from build123d import *

# Parameters (mm, degrees)
SKETCH_1_W          = 15.2
SKETCH_1_H          = 25
EXTRUDE_1_DEPTH     = 3
EXTRUDE_3_DEPTH     = 10
EXTRUDE_4_DEPTH     = 25
CUT_EXTRUDE_1_DEPTH = 18
FILLET_2_R          = 2
CHAMFER_1_SIZE      = 1
CHAMFER_2_SIZE      = 0.4


with BuildPart() as part:
    # 草图1 → 凸台-拉伸1 (new body)
    with BuildSketch(Plane(origin=(0, 0, 0), x_dir=(1, 0, 0), z_dir=(0, 1, 0))):
        Rectangle(SKETCH_1_W, SKETCH_1_H)
    extrude(amount=EXTRUDE_1_DEPTH)

    # 草图4 → 凸台-拉伸3 (add)
    with BuildSketch(Plane.ZY.offset(7.6)):
        Polygon((-12.5, -15), (-12.5, 3), (12.5, 3), (12.5, 0), align=None)
    extrude_3 = extrude(amount=EXTRUDE_3_DEPTH)

    # 镜向4: 凸台-拉伸3 across plane
    add(extrude_3.mirror(Plane(origin=(0, 0, 0), x_dir=(0, 0, 1), z_dir=(1, 0, 0))))

    # 草图5 → 凸台-拉伸4 (add)
    with BuildSketch(Plane(origin=(0, 0, -12.5), x_dir=(-1, 0, 0), z_dir=(0, 0, -1))):
        Polygon((7.6, 0), (7.6, -15), (17.6, -15), (17.6, 3), (-17.6, 3), (-17.6, -15), (-7.6, -15), (-7.6, 0), align=None)
    extrude(amount=EXTRUDE_4_DEPTH)

    # 草图6 → 切除-拉伸1 (cut)
    with BuildSketch(Plane(origin=(0, 3, 0), x_dir=(1, 0, 0), z_dir=(0, 1, 0))):
        Polygon((14.072075922, 37.6), (10.927924078, 37.6), (9.861257411, 34.4), (15.138742589, 34.4), align=None)
        Polygon((-14.072075922, 37.6), (-15.138742589, 34.4), (-9.861257411, 34.4), (-10.927924078, 37.6), align=None)
    extrude(amount=-CUT_EXTRUDE_1_DEPTH, mode=Mode.SUBTRACT)

    # 圆角2
    fillet_2_edges = [part.edges().sort_by_distance(p)[0] for p in [
        (-12.6, -15, -12.5),
        (12.6, -15, -12.5),
    ]]
    fillet(fillet_2_edges, radius=FILLET_2_R)

    # 倒角1
    chamfer_1_edges = [part.edges().sort_by_distance(p)[0] for p in [
        (-7.6, -7.357492926, 0.23751179),
        (-17.6, -7.357492926, 0.23751179),
        (-7.6, -14.927429856, -12.520100766),
        (-17.6, -14.927429856, -12.520100766),
        (7.6, -7.357492926, 0.23751179),
        (7.6, -14.927429856, -12.520100766),
        (17.6, -7.357492926, 0.23751179),
        (17.6, -14.927429856, -12.520100766),
        (-17.6, 1.5, 12.5),
        (-17.6, 3, -12.5),
        (17.6, 3, -12.5),
        (17.6, 1.5, 12.5),
        (7.6, -15, -25.276983965),
        (-7.6, -15, -25.276983965),
        (-17.6, -15, -25.276983965),
        (17.6, -15, -25.276983965),
        (7.6, -7.5, -37.5),
        (-7.6, -7.5, -37.5),
        (-17.6, -6, -37.5),
        (17.6, -6, -37.5),
    ]]
    chamfer(chamfer_1_edges, length=CHAMFER_1_SIZE)

    # 倒角2
    chamfer_2_edges = [part.edges().sort_by_distance(p)[0] for p in [
        (10.377924078, 3, -35.95),
        (12.5, 3, -34.4),
        (14.622075922, 3, -35.95),
        (14.622075922, -15, -35.95),
        (12.5, -15, -34.4),
        (10.377924078, -15, -35.95),
        (-14.622075922, 3, -35.95),
        (-12.5, 3, -34.4),
        (-10.377924078, 3, -35.95),
        (-10.377924078, -15, -35.95),
        (-12.5, -15, -34.4),
        (-14.622075922, -15, -35.95),
    ]]
    chamfer(chamfer_2_edges, length=CHAMFER_2_SIZE)


solid = part.part
Design review of the part built by this model. Coordinates are the model's own, in mm. A direction names the side the tool comes from. Give positions to 0.01 mm unless a question says otherwise; leave off trailing zeros. Write each loop counter-clockwise with the first axis right and the second up, starting at its lowest first coordinate (ties: lowest second). Pieces come first, ordered by that corner, then holes. Notation, with made-up numbers: M 80,59 L 103,59 A16 cw 103,80 Z; hole C 21,-7.5 d3. An arc over 180 degrees is marked long. Answer as a JSON object with one key per item and string values. Group by question number.
1) Mouldability with a two-part tool opening along X and no side actions: class faces 1 (the face through (14.911, -14.803, -35.726)), 2 (the face through (-17.1, -6.1, -37)), 3 (the face through (0, 2, -37.5)) as released by +X, released by -X, zero draft, split by the parting line, or undercut.
2) For line 1 along X through (y, z) = (-8.5, -11); line 2 along Y through (x, z) = (9, -3); line 3 along Y through (x, z) = (-1, -21.5), list the stretches that pass through material, from the lowest coordinate up.
3) We need section C-C (y = 1.25). Give the boundary of the cut face in (x, z).
4) We need section A-A (y = -9.25). Give the boundary of the cut face in (x, z), and give its area (3 significant figures).
5) Tool access review of faces 4 (the face through (-14.89, -14.8, -35.78)), 5 (the face through (-13, -6, -34.4)), 6 (the face through (8.1, -14.5, -25.1)): name each direction out of +Z, -Z, +X, -X, +Y, -Y from which nothing blocks a thin tool from reaching the whole face with its end or side.
6) We need section B-B (z = -32). Give the boundary of the cut face in (x, y), and give its area (3 significant figures).
7) Clearance check with flat-ended pins moving along their axes: pin 1 Ø19 at (x, z) = (1, -21.5) entering from -Y; pin 2 Ø8 at (y, z) = (-11, 1.5) entering from +X; pin 3 Ø4 at (x, z) = (-0.5, 4) entering from -Y; pin 4 Ø4 at (x, y) = (8, -3.5) entering from +Z. State where each tip first meets the part, or that it passes through.
8) We need section D-D (x = 13.5). Give the boundary of the cut face in (y, z), and give its area (3 significant figures).
Answer key:
{
 "1": {"face 1": "undercut", "face 2": "released by -X", "face 3": "zero draft"},
 "2": {"line 1": "x = -17.6 to -7.6, 7.6 to 17.6", "line 2": "y = -9.3 to 3", "line 3": "y = 0 to 3"},
 "3": {"outline": "M -17.6,-36.5 L -16.6,-37.5 L -14.11,-37.5 L -15.14,-34.4 L -9.86,-34.4 L -10.89,-37.5 L 10.89,-37.5 L 9.86,-34.4 L 15.14,-34.4 L 14.11,-37.5 L 16.6,-37.5 L 17.6,-36.5 L 17.6,11.5 L 16.6,12.5 L -16.6,12.5 L -17.6,11.5 Z"},
 "4": {"outline": "M -17.6,-36.5 L -16.6,-37.5 L -14.11,-37.5 L -15.14,-34.4 L -9.86,-34.4 L -10.89,-37.5 L -8.6,-37.5 L -7.6,-36.5 L -7.6,-4.86 L -8.6,-2.92 L -16.6,-2.92 L -17.6,-4.86 Z; M 7.6,-36.5 L 8.6,-37.5 L 10.89,-37.5 L 9.86,-34.4 L 15.14,-34.4 L 14.11,-37.5 L 16.6,-37.5 L 17.6,-36.5 L 17.6,-4.86 L 16.6,-2.92 L 8.6,-2.92 L 7.6,-4.86 Z", "area": "659 mm²"},
 "5": {"face 4": "-Y", "face 5": "+Y, -Y", "face 6": "+Z, -Z, -Y"},
 "6": {"outline": "M -17.6,-14 L -16.6,-15 L -8.6,-15 L -7.6,-14 L -7.6,0 L 7.6,0 L 7.6,-14 L 8.6,-15 L 16.6,-15 L 17.6,-14 L 17.6,2 L 16.6,3 L -16.6,3 L -17.6,2 Z", "area": "403 mm²"},
 "7": {"pin 1": "stops at y = -15", "pin 2": "stops at x = 16.83", "pin 3": "stops at y = 0", "pin 4": "stops at z = 9.85"},
 "8": {"outline": "M -15,-34 L -14.6,-34.4 L 2.6,-34.4 L 3,-34 L 3,12.5 L 0,12.5 L -14.71,-12.02 A2 ccw -15,-13.05 Z", "area": "657 mm²"}
}
